Autodesk Inventor part; units mm, degrees
ref_plane "YZ Plane" through (0, 0, 0) normal (1, 0, 0) x (0, 1, 0)
ref_plane "XZ Plane" through (0, 0, 0) normal (0, 1, 0) x (-1, 0, 0)
ref_plane "XY Plane" through (0, 0, 0) normal (0, 0, 1) x (1, 0, 0)
sketch "Sketch1" plane through (0, 0, 0) normal (0, 0, 1) x (1, 0, 0)
  line L0 (0, 0) -> (41.275, 0)
  line L1 (41.275, 0) -> (41.275, 101.6)
  line L2 (41.275, 101.6) -> (0, 101.6)
  line L3 (0, 101.6) -> (0, 0)
  dimension "d0" = 101.6
  dimension "d1" = 41.275
extrude "Plate1" add sketch "Sketch1" along normal blind 2.032
sketch "Sketch2" plane through (39.243, 101.6, 0) normal (1, 0, 0) x (0, 1, 0)
  line L0 (-101.6, 0) -> (0, 0)
  line L1 (0, 0) -> (0, 66.04)
  line L2 (0, 66.04) -> (-101.6, 66.04)
  line L3 (-101.6, 66.04) -> (-101.6, 0)
edge flange "Flange1" height 66.04 angle 90 thickness 2.032 bend radius 1.27 thickness toward (1, 0, 0) relief tear relief width 2.032 relief depth 1.016 edges at (41.275, 50.8, 2.032) wall of the first edge with corners at (39.243, 0, 0) (39.243, 101.6, 0) (39.243, 101.6, 66.04) (39.243, 0, 66.04)
bend "Bend1"
corner "Corner1"
sketch "Sketch3" plane through (0, 0, 2.032) normal (0, 0, 1) x (1, 0, 0)
  line L0 (0, 0) -> (0, 101.6)
  line L1 (0, 101.6) -> (37.973, 101.6)
  point P0 (6.35, 95.25)
  point P1 (6.35, 57.15)
  point P2 (19.05, 95.25)
  point P3 (31.75, 95.25)
  point P4 (19.05, 57.15)
  dimension "d13" = 6.35
  dimension "d14" = 6.35
  dimension "d15" = 38.1
  dimension "d16" = 12.7
  dimension "d17" = 12.7
hole "Hole1" at (6.35, 95.25, 2.032) at (6.35, 57.15, 2.032) at (19.05, 95.25, 2.032) at (31.75, 95.25, 2.032) at (19.05, 57.15, 2.032) direction (0, 0, -1) diameter 4.8514 end through all
sketch "Sketch4" plane through (0, 0, 2.032) normal (0, 0, 1) x (1, 0, 0)
  line L0 (0, 101.6) -> (37.973, 101.6)
  line L1 (0, 0) -> (0, 101.6)
  point P0 (12.7, 26.6446)
  dimension "d25" = 74.9554
  dimension "d26" = 12.7
hole "Hole2" at (12.7, 26.6446, 2.032) direction (0, 0, -1) diameter 7.9375 end through all
sketch "Sketch5" plane through (0, 0, 2.032) normal (0, 0, 1) x (1, 0, 0)
  circle A0 centre (12.7, 26.6446) radius 3.9687
  arc A1 (5.6431, 25.4938) -> (19.3942, 24.1322) centre (12.7, 26.6446) ccw
  line L0 (37.973, 101.6) -> (37.973, 0)
  line L1 (0, 101.6) -> (37.973, 101.6)
  line L2 (39.243, 101.6) -> (39.243, 0)
  line L3 (39.243, 60.0989) -> (32.893, 60.0989)
  line L4 (32.893, 60.0989) -> (19.3942, 24.1322)
  line L5 (0, 60.0989) -> (5.6431, 25.4938)
  line L6 (0, 0) -> (0, 101.6)
  line L7 (37.973, 0) -> (0, 0)
  line L8 (0, 60.0989) -> (0, 0)
  line L9 (0, 0) -> (39.243, 0)
  dimension "d34" = 14.3002
  dimension "d37" = 6.35
  dimension "d38" = 41.5011
extrude "Extrusion1" cut sketch "Sketch5" against normal through all contours A1 L4 L3 L0 L7 L6 L5 | L3 L2 L9 L0
sketch "Sketch6" plane through (39.243, 0, 66.04) normal (-1, 0, 0) x (0, 0, 1)
  line L0 (-66.04, 101.6) -> (-66.04, 60.0989)
  line L1 (-62.738, 101.6) -> (0, 101.6)
  point P0 (-66.04, 0)
  point P1 (-15.24, 40.7924)
  dimension "d41" = 50.8
  dimension "d42" = 60.8076
hole "Hole3" at (39.243, 40.7924, 50.8) direction (1, 0, 0) diameter 22.225 end through all
sketch "Sketch7" plane through (39.243, 0, 66.04) normal (-1, 0, 0) x (0, 0, 1)
  line L0 (0, 0) -> (0, 101.6)
  line L1 (0, 25.4) -> (-31.75, 25.4)
  line L2 (-62.738, 101.6) -> (0, 101.6)
  line L3 (-64.008, 60.0989) -> (-65.786, 60.0989)
  line L4 (-65.786, 60.0989) -> (-46.736, 60.0989)
  line L5 (-31.75, 25.4) -> (-46.736, 60.0989)
  line L6 (0, 25.4) -> (0, 0)
  line L7 (-65.786, 0) -> (-65.786, 60.0989)
  line L8 (-65.786, 0) -> (-65.786, 60.0989)
  line L9 (0, 0) -> (-65.786, 0)
  point P0 (-66.04, 0)
  dimension "d50" = 76.2
  dimension "d51" = 31.75
  dimension "d54" = 19.05
extrude "Extrusion2" cut sketch "Sketch7" against normal blind 6.35 and the other way blind 6.35
fillet "Fillet1" radius 12.7 1 edges at (40.259, 60.0989, 19.304)
sketch "Sketch8" plane through (39.243, 101.6, 3.302) normal (-1, 0, 0) x (0, 0, 1)
  line L0 (62.738, -76.2) -> (62.738, 0)
  line L1 (62.738, -50.8) -> (62.738, 0)
  line L2 (62.738, 0) -> (6.223, 0)
  line L3 (62.738, 0) -> (0, 0)
  line L4 (62.738, -50.8) -> (6.223, 0)
  line L5 (-3.302, 0) -> (-3.302, -41.5011)
  point P0 (-3.302, -101.6)
  dimension "d60" = 50.8
  dimension "d61" = 9.525
extrude "Extrusion3" cut sketch "Sketch8" against normal through all
equation "\"d23\" = Thickness"
equation "\"d32\" = Thickness"
equation "\"d48\" = Thickness"
equation "\"d2\" = Thickness"
equation "\"d3\" = BendReliefWidth"
equation "\"d4\" = BendReliefDepth"
equation "\"d5\" = MinimumRemnant"
equation "\"d6\" = TransitionRadius"
equation "\"d9\" = BendRadius"
equation "\"d10\" = CornerReliefSize"
equation "\"d11\" = GapSize"
equation "\"d12\" = JacobiRadiusSize"
equation "\"BendReliefWidth\" = Thickness"
equation "\"BendReliefDepth\" = 0.5 * Thickness"
equation "\"CornerReliefSize\" = 4 * Thickness"
equation "\"MinimumRemnant\" = 2 * Thickness"
equation "\"TransitionRadius\" = BendRadius"
equation "\"JacobiRadiusSize\" = BendRadius"
equation "\"GapSize\" = Thickness"
properties part number "Roller bracket" material "Aluminum 6061"
Design review of the part built by this model. Coordinates are the model's own, in mm. Coordinates: 2 decimals unless noted, no trailing zeros. Loops run counter-clockwise (first coordinate to the right, second up) from the corner with the lowest first, then second, coordinate; pieces in that order, holes last. Notation, with made-up numbers: (-11, 42.25) - (16, 42.25) arc R22 ccw to (16, 70.25) - close; hole circle Ø11 at (24, 54). An arc over 180 degrees is marked (long way). Use CSV: the item, a comma, the result in double quotes. Start each with the question number.
1. Add section B-B on y = 57.15. Give the boundary of the cut face in (x, z) (3 decimals), plus the area to 3 significant figures.
2. Clearance check with flat-ended pins moving along their axes: pin 1 (4 mm diameter, centred on x = 32, y = 79.5, fed in from +Z); pin 2 (1.6 mm diameter, centred on x = 40, z = 47.5, fed in from -Y); pin 3 (19 mm diameter, centred on y = 63.5, z = 27.5, fed in from -X). State where each tip first meets the part, or that it passes through.
3. To check wall thickness, follow probe 1 along X at (y, z) = (57, 1); probe 2 along Y at (x, z) = (6.35, 0.6); probe 3 along X at (y, z) = (95.25, 1.25). State the ranges of each line that lie inside material, in increasing order.
4. Add section C-C on z = 50.8. Give the boundary of the cut face in (x, y) (3 decimals).
5. Add section D-D on y = 71. Give the boundary of the cut face in (x, z) (1 decimal), plus the area to 3 significant figures.
6. Add section A-A on x = 12.7. Give the boundary of the cut face in (y, z), plus the area to 3 significant figures.
7. Mouldability with a two-part tool opening along Y and no side actions: class faces 1 (the cylindrical face through (19.98, 54.91, 1)), 2 (the flat face through (0, 81, 1)), 3 (the flat face through (40, 60.099, 4)) as released by +Y, released by -Y, zero draft, split by the parting line, or undercut.
Resolved:
1,outline,"(0.481, 0) - (3.924, 0) - (3.924, 2.032) - (0.481, 2.032) - close; (8.776, 0) - (16.624, 0) - (16.624, 2.032) - (8.776, 2.032) - close; (21.476, 0) - (31.786, 0) - (31.786, 2.032) - (21.476, 2.032) - close; (39.243, 19.092) - (41.275, 19.092) - (41.275, 58.976) - (39.243, 58.976) - close"
1,area,"125 mm2"
2,pin 1,"z = 2.03"
2,pin 2,"y = 25.4"
2,pin 3,"x = 39.24"
3,probe 1,"0.51 to 3.93, 8.77 to 16.63, 21.47 to 31.73"
3,probe 2,"23.36 to 54.72, 59.58 to 92.82, 97.68 to 101.6"
3,probe 3,"0 to 3.92, 8.78 to 16.62, 21.48 to 29.32, 34.18 to 40.56"
4,outline,"(39.243, 25.4) - (41.275, 25.4) - (41.275, 29.68) - (39.243, 29.68) - close; (39.243, 51.905) - (41.275, 51.905) - (41.275, 64.499) - (39.243, 64.499) - close"
5,outline,"(0, 0) - (38, 0) arc R3.3 ccw to (41.3, 3.3) - (41.3, 43.6) - (39.2, 43.6) - (39.2, 3.3) arc R1.3 cw to (38, 2) - (0, 2) - close"
5,area,"166 mm2"
6,outline,"(19.49, 0) - (22.68, 0) - (22.68, 2.03) - (19.49, 2.03) - close; (30.61, 0) - (101.6, 0) - (101.6, 2.03) - (30.61, 2.03) - close"
6,area,"151 mm2"
7,face 1,"undercut"
7,face 2,"zero draft"
7,face 3,"released by -Y"
